```python
from build123d import *

# Parameters (mm, degrees)
F0_R          = 11
F0_R_2        = 6
F1_DEPTH      = 12
F2_SIZE       = 0.5
F3_R          = 3
F4_DEPTH      = 25
F4_DEPTH_BACK = 25


with BuildPart() as f1:
    # F0 (on Front) → F1 (new body)
    with BuildSketch(Plane.XZ):
        Circle(F0_R)
        Circle(F0_R_2, mode=Mode.SUBTRACT)
    extrude(amount=F1_DEPTH)

    # F2
    f2_edges = [f1.edges().sort_by_distance(p)[0] for p in [
        (-11, -12, 0),
    ]]
    chamfer(f2_edges, length=F2_SIZE)

    # F3 (on Top) → F4 (cut, two sides)
    with BuildSketch(Plane.XY) as f4_sk:
        with Locations((0, -6)):
            Circle(F3_R)
    extrude(amount=F4_DEPTH, mode=Mode.SUBTRACT)
    extrude(f4_sk.sketch, amount=-F4_DEPTH_BACK, mode=Mode.SUBTRACT)


solid = f1.part
```
Here's how the part is built. I have some questions about the finished solid (model axes, mm). Give positions to 0.01 mm unless a question says otherwise; leave off trailing zeros. Loops run counter-clockwise (first coordinate to the right, second up) from the corner with the lowest first, then second, coordinate; pieces in that order, holes last. Notation, with made-up numbers: (-12, 67) -> (27, 67) arc R18 ccw to (27, 72) -> close; hole circle Ø3 at (13.5, 23.25). An arc over 180 degrees is marked (long way). Use one line per item in the form item = value. Start each with the question number.
1) Imagine slicing it at C-C (y = -10.75). Please give me the cut outline in (x, z), then the cut area to 3 significant figures.
2) Imagine slicing it at A-A (z = 0). Please give me the cut outline in (x, y), then the cut area to 3 significant figures.
3) Thinking about a two-plate mould opening in Z: for faces 1 (the face through (10.161, -5.67, -4.213)), 2 (the face through (5.54, -5.92, -2.3)), 3 (the face through (5, -12, -5)), which applies, +Z half, -Z half, draft (parallel to the pull), parting line (faces both ways), or undercut?
4) Imagine slicing it at B-B (x = 0). Please give me the cut outline in (y, z).
5) Imagine slicing it at D-D (y = -6). Please give me the cut outline in (x, z).
6) For P1, Ø1.5, axis at y = -10.5, z = 2, coming from the -X side; P2, Ø5, axis at x = 8.5, y = -1.5, coming from the -Z side; P3, Ø6, axis at y = -6, z = -9, coming from the -X side, each with a flat end and sliding along its axis, tell me the tip position at first contact or that it passes through.
7) Please list where these lines run through material, in increasing order: line 1 along Y through (x, z) = (0, -6.4); line 2 along Z through (x, y) = (-2.5, -2.25); line 3 along X through (y, z) = (-9.5, 3.5).
Check values:
q1.outline = circle Ø22 at (0, 0); hole circle Ø12 at (0, 0)
q1.area = 267 mm^2
q2.outline = (-11, -11.5) -> (-10.5, -12) -> (-6, -12) -> (-6, 0) -> (-11, 0) -> close; (6, -12) -> (10.5, -12) -> (11, -11.5) -> (11, 0) -> (6, 0) -> close
q2.area = 120 mm^2
q3.face_1 = parting line
q3.face_2 = undercut
q3.face_3 = draft
q4.outline = (-12, -10.5) -> (-11.5, -11) -> (-9, -11) -> (-9, -6) -> (-12, -6) -> close; (-12, 6) -> (-9, 6) -> (-9, 11) -> (-11.5, 11) -> (-12, 10.5) -> close; (-3, -11) -> (0, -11) -> (0, -6) -> (-3, -6) -> close; (-3, 6) -> (0, 6) -> (0, 11) -> (-3, 11) -> close
q5.outline = (-3, -10.58) -> (-3, -5.2) arc R6 cw to (-3, 5.2) -> (-3, 10.58) arc R11 ccw to start; (3, -10.58) arc R11 ccw to (3, 10.58) -> (3, 5.2) arc R6 cw to (3, -5.2) -> close
q6.P1 = -10.93
q6.P2 = -9.22
q6.P3 = -9.22
q7.line_1 = -12 to -9, -3 to 0
q7.line_2 = -10.71 to -5.45, 5.45 to 10.71
q7.line_3 = -10.43 to -4.87, 4.87 to 10.43
